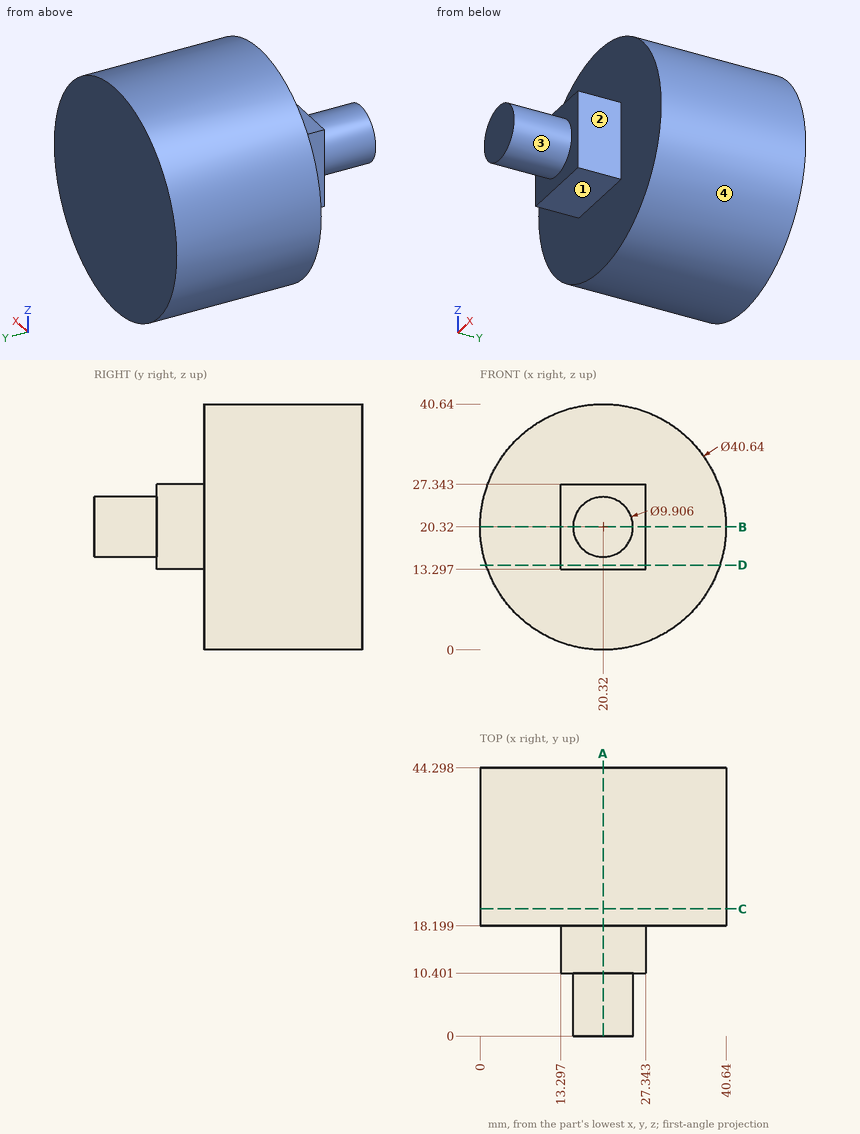
Drawing for the job (mm, zero at the part's lowest x, y, z). A direction names the side the tool comes from. Round coordinates to 2 decimals unless told otherwise and drop trailing zeros. Write each loop counter-clockwise with the first axis right and the second up, starting at its lowest first coordinate (ties: lowest second). Pieces come first, ordered by that corner, then holes. Notation, with made-up numbers: M -13,79.25 L 31,79.25 A29 ccw 31,99.25 Z; hole C 39,-2 d8. An arc over 180 degrees is marked long. Put each result on its own line as item: value.
Item 1: Probe L1, parallel to Y at x = 35, z = 13.5; L2, parallel to Y at x = 16, z = 17; L3, parallel to Z at x = 20, y = 16. List the from-to ranges inside material, lowest first. Write a range as from..to.
Responses:
L1: 18.2..44.3
L2: 10.4..44.3
L3: 13.3..27.34
Item 2: Flat gauge pins, fed straight in: P1, Ø12, axis at y = 18.5, z = 18, coming from the +X side; P2, Ø12, axis at x = 19.5, y = 6, coming from the +Z side; P3, Ø2.5, axis at x = 23.5, y = 15.5, coming from the -Z side; P4, Ø1, axis at y = 11, z = 11, coming from the +X side. Where does each tip first touch, or does it go through?
Responses:
P1: x = 40.64
P2: z = 27.34
P3: z = 13.3
P4: through
Item 3: Cut at B-B (z = 20.32). List the corners of the cut face in (x, y), and give its area (3 significant figures).
Responses:
outline: M 0,18.2 L 13.3,18.2 L 13.3,10.4 L 15.37,10.4 L 15.37,0 L 25.27,0 L 25.27,10.4 L 27.34,10.4 L 27.34,18.2 L 40.64,18.2 L 40.64,44.3 L 0,44.3 Z
area: 1,270 mm²
Item 4: Cut at D-D (z = 14). List the corners of the cut face in (x, y), and give its area (3 significant figures).
Responses:
outline: M 1.01,18.2 L 13.3,18.2 L 13.3,10.4 L 27.34,10.4 L 27.34,18.2 L 39.63,18.2 L 39.63,44.3 L 1.01,44.3 Z
area: 1,120 mm²
Item 5: Cut at C-C (y = 21). List the corners of the cut face in (x, z).
Responses:
outline: C 20.32,20.32 d40.64
Item 6: Tool access for the marked faces 1, 2, 3 and 4: list every direction of +Z, -Z, +X, -X, +Y, -Y with a clear straight run to the whole face (end or side of a thin tool).
Responses:
face 1: -Z, +X, -X, -Y
face 2: +Z, -Z, +X, -Y
face 3: -Y
face 4: +Y, -Y
Item 7: Cut at A-A (x = 20.32). List the corners of the cut face in (y, z).
Responses:
outline: M 0,15.37 L 10.4,15.37 L 10.4,13.3 L 18.2,13.3 L 18.2,0 L 44.3,0 L 44.3,40.64 L 18.2,40.64 L 18.2,27.34 L 10.4,27.34 L 10.4,25.27 L 0,25.27 Z
